Design review of the part built by this model. Coordinates are the model's own, in mm. A direction names the side the tool comes from. Round coordinates to 2 decimals unless told otherwise and drop trailing zeros. Order: outer loops, then holes, each group sorted by start corner. A loop starts at its lowest first (then second) coordinate and runs counter-clockwise, first axis right, second up. Notation, with made-up numbers: M 35,11 L 89,11 A23 ccw 89,28 Z; hole C 12.5,-5 d8. An arc over 180 degrees is marked long. Use a Markdown table: item, result. Add a question column.
(1) Take a section at C-C (z = 16). Write out the cut boundary in (x, y).
(2) The part is to be moulded in two halves that separate along X. For faces 4 (the face through (0, 0, 2)), 5 (the face through (-1.062, -4.783, 2.169)), 6 (the face through (-2, 2, 14.4)), say which applies: released by +X, released by -X, zero draft, split by the parting line, or undercut.
(3) Take a section at B-B (x = 0.5). Write out the cut boundary in (y, z).
(4) Take a section at D-D (y = 2). Write out the cut boundary in (x, z).
(5) To check wall thickness, follow probe 1 along Z at (x, y) = (4, -2); probe 2 along Z at (x, y) = (-0.5, -2.5); probe 3 along Y at (x, z) = (1.5, 18.5). State the ranges of each line that lie inside material, in increasing order. Write a range as from..to.
(6) For pin 1 (3 mm diameter, centred on y = 3, z = 2.5, fed in from -X); pin 2 (3 mm diameter, centred on x = 0.5, y = 1, fed in from -Z); pin 3 (1 mm diameter, centred on x = 3.5, z = 15, fed in from -Y); pin 4 (5 mm diameter, centred on x = 0, z = 11, fed in from -Y), all flat-tipped, find the tip position at first contact; note any pin that passes through.
(7) Machinability: for faces 1 (the face through (0, 0, 24.1)), 2 (the face through (-3, 0, 9)), 3 (the face through (1.5, 0, 1)), which of the approach directions +Z, -Z, +X, -X, +Y, -Y give a long, thin tool a straight path to every point of the face, cutting with its end or side? Answer none if there is none.
(8) Take a section at A-A (y = 0). Write out the cut boundary in (x, z).
```python
from build123d import *

# Parameters (mm, degrees)
SKETCH_1_R          = 4.9
EXTRUDE_1_DEPTH     = 4.4
SKETCH_2_R          = 3
EXTRUDE_2_DEPTH     = 10
SKETCH_3_R          = 2.5
EXTRUDE_3_DEPTH     = 9.7
CUT_EXTRUDE_1_DEPTH = 2


with BuildPart() as part:
    # 草图1 → 凸台-拉伸1 (new body)
    with BuildSketch(Plane.XY):
        Circle(SKETCH_1_R)
    extrude(amount=EXTRUDE_1_DEPTH)

    # 草图2 → 凸台-拉伸2 (add)
    with BuildSketch(Plane.XY.offset(4.4)):
        Circle(SKETCH_2_R)
    extrude(amount=EXTRUDE_2_DEPTH)

    # 草图3 → 凸台-拉伸3 (add)
    with BuildSketch(Plane.XY.offset(14.4)):
        Circle(SKETCH_3_R)
    extrude(amount=EXTRUDE_3_DEPTH)

    # 草图4 → 切除-拉伸1 (cut)
    with BuildSketch(Plane(origin=(0, 0, 0), x_dir=(-1, 0, 0), z_dir=(0, 0, -1))):
        Polygon((0, 1.732050808), (-1.5, 0.866025404), (-1.5, -0.866025404), (0, -1.732050808), (1.5, -0.866025404), (1.5, 0.866025404), align=None)
    extrude(amount=-CUT_EXTRUDE_1_DEPTH, mode=Mode.SUBTRACT)


solid = part.part
```
Verdict:
| question | item | result |
|---|---|---|
| 1 | outline | C 0,0 d5 |
| 2 | face 4 | undercut |
| 2 | face 5 | split by the parting line |
| 2 | face 6 | zero draft |
| 3 | outline | M -4.87,0 L -1.44,0 L -1.44,2 L 1.44,2 L 1.44,0 L 4.87,0 L 4.87,4.4 L 2.96,4.4 L 2.96,14.4 L 2.45,14.4 L 2.45,24.1 L -2.45,24.1 L -2.45,14.4 L -2.96,14.4 L -2.96,4.4 L -4.87,4.4 Z |
| 4 | outline | M -4.47,0 L 4.47,0 L 4.47,4.4 L 2.24,4.4 L 2.24,14.4 L 1.5,14.4 L 1.5,24.1 L -1.5,24.1 L -1.5,14.4 L -2.24,14.4 L -2.24,4.4 L -4.47,4.4 Z |
| 5 | probe 1 | z = 0..4.4 |
| 5 | probe 2 | z = 0..14.4 |
| 5 | probe 3 | y = -2..2 |
| 6 | pin 1 | stops at x = -4.66 |
| 6 | pin 2 | stops at z = 0 |
| 6 | pin 3 | passes through |
| 6 | pin 4 | stops at y = -3 |
| 7 | face 1 | +Z, +X, -X, +Y, -Y |
| 7 | face 2 | +Z |
| 7 | face 3 | -Z |
| 8 | outline | M -4.9,0 L -1.5,0 L -1.5,2 L 1.5,2 L 1.5,0 L 4.9,0 L 4.9,4.4 L 3,4.4 L 3,14.4 L 2.5,14.4 L 2.5,24.1 L -2.5,24.1 L -2.5,14.4 L -3,14.4 L -3,4.4 L -4.9,4.4 Z |
